```python
from build123d import *

# Parameters (mm, degrees)
F1_DEPTH = 25
F2_R     = 9.1373758173
F3_DEPTH = 18.8
F6_D     = 5.5
F9_D     = 13.2


with BuildPart() as f1:
    # F0 (on Front) → F1 (new body)
    with BuildSketch(Plane.XZ):
        with BuildLine():
            Line((20.4618610442, 41.5807515383), (-41.8623387814, 41.5807515383))
            ThreePointArc((-41.8623387814, 41.5807515383), (-42.1671038517, 59.9239812985), (-58.3820044994, 51.3423755765))
            ThreePointArc((-58.3820044994, 51.3423755765), (-73.5517436915, 40.4678527546), (-55.0029836595, 38.3894555271))
            Line((-55.0029836595, 38.3894555271), (-60.2592416108, 28.2523836941))
            Line((-60.2592416108, 28.2523836941), (-41.2991680205, 24.8733609915))
            Line((-41.2991680205, 24.8733609915), (-56.8802170455, 8.5414182395))
            Line((-56.8802170455, 8.5414182395), (-36.9815267622, 8.5414182395))
            Line((-36.9815267622, 8.5414182395), (-28.8509290056, 26.3923599584))
            Line((-28.8509290056, 26.3923599584), (-17.4582842737, 28.2523836941))
            Line((-17.4582842737, 28.2523836941), (-14.4547084346, 9.8554827273))
            Line((-14.4547084346, 9.8554827273), (11.6388564929, 9.8554827273))
            Line((11.6388564929, 9.8554827273), (33.7902270257, -11.5449940786))
            Line((33.7902270257, -11.5449940786), (20.4618610442, 41.5807515383))
        make_face()
    extrude(amount=F1_DEPTH)

    # F2 (on face) → F3 (join)
    with BuildSketch(Plane.XY.offset(41.5807515383)):
        with Locations((-12.0476996526, -13.8280903921)):
            Circle(F2_R)
    extrude(amount=F3_DEPTH)

    # F6 (through all)
    with Locations(Plane(origin=(29.0643953622, 0, 7.2917733939), x_dir=(0, 1, 0), z_dir=(0.9699405616, 0, 0.2433419547))):
        with Locations((-7.6085178865, 11.3008453181)):
            Hole(F6_D / 2)

    # F9 (through all)
    with Locations(Plane(origin=(0, 0, 0), x_dir=(-1, 0, 0), z_dir=(0, 1, 0))):
        with Locations((-7.8541710973, 19.9797544628)):
            Hole(F9_D / 2)


solid = f1.part
```
Model file for the job. Use its own axes, mm. A direction names the side the tool comes from. Round coordinates to 2 decimals unless told otherwise and drop trailing zeros. Write each loop counter-clockwise with the first axis right and the second up, starting at its lowest first coordinate (ties: lowest second). Pieces come first, ordered by that corner, then holes. Notation, with made-up numbers: (12.5, 3.5) - (20.5, 3.5) arc R26 ccw to (20.5, 18.5) - close; hole circle Ø7 at (53.25, 88). An arc over 180 degrees is marked (long way). One line per item, written item: value.
(1) Cut at D-D, the plane y = -7.25. Give the cut face in (x, z) (1 decimal).
Values follow:
outline: (-60.3, 28.3) - (-41.3, 24.9) - (-56.9, 8.5) - (-37, 8.5) - (-28.9, 26.4) - (-17.5, 28.3) - (-14.6, 10.8) - (3.2, 15.3) arc R6.6 cw (long way) to (14.2, 18) - (25.7, 20.9) - (20.5, 41.6) - (-5.7, 41.6) - (-5.7, 60.4) - (-18.4, 60.4) - (-18.4, 41.6) - (-41.9, 41.6) arc R10.8 ccw (long way) to (-58.4, 51.3) arc R10 ccw (long way) to (-55, 38.4) - close; (4, 9.9) - (11.6, 9.9) - (33.8, -11.5) - (27, 15.6) - close
(2) Wall check: probe 1 along Z at (x, y) = (-64.5, -15); probe 2 along Z at (x, y) = (-41, -16.25); probe 3 along Z at (x, y) = (-50, -15). Give the ranges that are in metal, low to high.
Values follow:
probe 1: z = 33.01 to 52.97
probe 2: z = 8.54 to 41.58, 42.19 to 59.13
probe 3: z = 8.54 to 15.75, 26.42 to 61.16
(3) Cut at C-C, the plane y = -18.75. Give the cut face in (x, z) (3 decimals).
Values follow:
outline: (-60.259, 28.252) - (-41.299, 24.873) - (-56.88, 8.541) - (-36.982, 8.541) - (-28.851, 26.392) - (-17.458, 28.252) - (-14.455, 9.855) - (11.639, 9.855) - (33.79, -11.545) - (20.462, 41.581) - (-4.349, 41.581) - (-4.349, 60.381) - (-19.746, 60.381) - (-19.746, 41.581) - (-41.862, 41.581) arc R10.762 ccw (long way) to (-58.382, 51.342) arc R9.997 ccw (long way) to (-55.003, 38.389) - close; hole circle Ø13.2 at (7.854, 19.98)
(4) Cut at A-A, the plane z = 35. Give the cut face in (x, y).
Values follow:
outline: (-69.89, -25) - (-57.87, -25) - (-57.87, 0) - (-69.89, 0) - close; (-56.76, -25) - (22.11, -25) - (22.11, 0) - (-56.76, 0) - close
(5) Drop flat-ended pins along their axis: P1, Ø1, axis at y = -7, z = 24, coming from the -X side; P2, Ø2, axis at x = -61.5, y = -7.5, coming from the +Z side; P3, Ø5, axis at y = -8, z = 35.5, coming from the -X side; P4, Ø3, axis at x = -58, z = 6, coming from the +Y side (1 decimal). Give the stop position or say it passes through.
Values follow:
P1: stops at x = -42.61
P2: stops at z = 52.89
P3: stops at x = -72.54
P4: passes through
(6) Cut at B-B, the plane x = -53. Give the cut face in (y, z), plus the area to 3 significant figures.
Values follow:
outline: (-25, 8.54) - (0, 8.54) - (0, 12.61) - (-25, 12.61) - close; (-25, 26.96) - (0, 26.96) - (0, 59.99) - (-25, 59.99) - close
area: 928 mm²
(7) Two-plate mould, pull along Z, no slides. Class faces 6 (the cylindrical face through (6.995, -12.675, 26.524)), 7 (the flat face through (22.559, -12.325, -0.695)), 8 (the cylindrical face through (-14.029, -22.748, 50.849)): pulls with the +Z half, pulls with the -Z half, needs draft (parallel to the pull), parting line crosses it, or undercut.
Values follow:
face 6: undercut
face 7: pulls with the -Z half
face 8: needs draft
(8) 3-axis set-ups, long thin cutter, end or side, ignore diameter. For faces 1 (the flat face through (-47, -12, 8.541)), 2 (the flat face through (-50.912, -12.325, 26.587)), 3 (the flat face through (-23.23, -12.32, 27.31)), 4 (the flat face through (-12, -14, 60.381)), 5 (the flat face through (-24, 0, 31)): which of +Z, -Z, +X, -X, +Y, -Y reach the whole face in a straight line?
Values follow:
face 1: -Z, -X, +Y, -Y
face 2: -X, +Y, -Y
face 3: -Z, +Y, -Y
face 4: +Z, +X, +Y, -Y
face 5: +Z, -Z, +X, -X, +Y
